Could you check a few things on this model? Use its own coordinates, in mm. A direction names the side the tool comes from. Coordinates: 2 decimals unless noted, no trailing zeros. Loops run counter-clockwise (first coordinate to the right, second up) from the corner with the lowest first, then second, coordinate; pieces in that order, holes last. Notation, with made-up numbers: (88.25, 37.25) - (117.25, 37.25) arc R16 ccw to (117.25, 65.25) - close; hole circle Ø1 at (-12, 43). An arc over 180 degrees is marked (long way). Use CSV: the item, a comma, the result in double quotes.
from build123d import *

# Parameters (mm, degrees)
BOSS_EXTRUDE1_START     = -26
SKETCH1_R               = 20
BOSS_EXTRUDE1_DEPTH     = 3
BOSS_EXTRUDE2_START     = -26
SKETCH2_W               = 20
SKETCH2_H               = 49
BOSS_EXTRUDE2_DEPTH     = 3
BOSS_EXTRUDE3_START     = -26
SKETCH3_W               = 3
SKETCH3_H               = 49
BOSS_EXTRUDE3_DEPTH     = 38
CUT_EXTRUDE1_DEPTH      = 52.730068626
CUT_EXTRUDE1_DEPTH_BACK = 52.730068626
SKETCH4_R               = 2.75
SKETCH4_R_2             = 0.8
CUT_EXTRUDE2_DEPTH      = 52.730068626
CUT_EXTRUDE2_DEPTH_BACK = 52.730068626
SKETCH5_R               = 1.725


with BuildPart() as part:
    # Sketch1 → Boss-Extrude1 (new body)
    with BuildSketch(Plane.XY.offset(BOSS_EXTRUDE1_START)):
        Circle(SKETCH1_R)
    extrude(amount=BOSS_EXTRUDE1_DEPTH)

    # Sketch2 → Boss-Extrude2 (add)
    with BuildSketch(Plane.XY.offset(BOSS_EXTRUDE2_START)):
        with Locations((10, -15.5)):
            Rectangle(SKETCH2_W, SKETCH2_H)
    extrude(amount=BOSS_EXTRUDE2_DEPTH)

    # Sketch3 → Boss-Extrude3 (add)
    with BuildSketch(Plane.XY.offset(BOSS_EXTRUDE3_START)):
        with Locations((18.5, -15.5)):
            Rectangle(SKETCH3_W, SKETCH3_H)
    extrude(amount=BOSS_EXTRUDE3_DEPTH)

    # Sketch4 → Cut-Extrude1 (cut, two sides: drawn at the far end of the back side and taken through both)
    with BuildSketch(Plane.XY.offset(-CUT_EXTRUDE1_DEPTH_BACK)):
        Circle(SKETCH4_R)
        with Locations((0, 6)):
            Circle(SKETCH4_R_2)
        with Locations((0, -6)):
            Circle(SKETCH4_R_2)
        with Locations((0, 17)):
            Circle(SKETCH4_R_2)
        with Locations((0, -17)):
            Circle(SKETCH4_R_2)
    extrude(amount=CUT_EXTRUDE1_DEPTH + CUT_EXTRUDE1_DEPTH_BACK, mode=Mode.SUBTRACT)

    # Sketch5 → Cut-Extrude2 (cut, two sides: drawn at the far end of the back side and taken through both)
    with BuildSketch(Plane(origin=(0, 0, 0), x_dir=(0, 0, -1), z_dir=(1, 0, 0)).offset(-CUT_EXTRUDE2_DEPTH_BACK)):
        with Locations((-6, -31)):
            Circle(SKETCH5_R)
        with Locations((6, -31)):
            Circle(SKETCH5_R)
    extrude(amount=CUT_EXTRUDE2_DEPTH + CUT_EXTRUDE2_DEPTH_BACK, mode=Mode.SUBTRACT)


solid = part.part
(1) Suppose I cut it at A-A (y = 0). Write out the boundary of the cut face in (x, z), plus the area to 4 significant figures.
Computed:
outline,"(-20, -26) - (-2.75, -26) - (-2.75, -23) - (-20, -23) - close; (2.75, -26) - (20, -26) - (20, 12) - (17, 12) - (17, -23) - (2.75, -23) - close"
area,"208.5 mm²"
(2) Thinking about a two-plate mould opening in Z: for faces 1 (the face through (4, -10, -26)), 2 (the face through (0.37, 16.29, -24.52)), 3 (the face through (18.479, -32.684, -5.626)), which applies, +Z half, -Z half, draft (parallel to the pull), parting line (faces both ways), or undercut?
Computed:
face 1,"-Z half"
face 2,"draft"
face 3,"undercut"
(3) Suppose I cut it at C-C (y = -31). Write out the boundary of the cut face in (x, z) (3 decimals), plus the area to 3 significant figures.
Computed:
outline,"(0, -26) - (20, -26) - (20, -7.725) - (17, -7.725) - (17, -23) - (0, -23) - close; (17, -4.275) - (20, -4.275) - (20, 4.275) - (17, 4.275) - close; (17, 7.725) - (20, 7.725) - (20, 12) - (17, 12) - close"
area,"144 mm²"
(4) Please list where these lines run through material, in increasing order: line 1 (Z direction, x = 18, y = -31) (3 decimals); line 2 (X direction, y = 0, z = -24); line 3 (Y direction, x = 18, z = -6) (3 decimals).
Computed:
line 1,"z = -26 to -7.725, -4.275 to 4.275, 7.725 to 12"
line 2,"x = -20 to -2.75, 2.75 to 20"
line 3,"y = -40 to -32.725, -29.275 to 9"
(5) Suppose I cut it at D-D (x = 16). Write out the boundary of the cut face in (y, z).
Computed:
outline,"(-40, -26) - (12, -26) - (12, -23) - (-40, -23) - close"
(6) Will these pins go through, and if not, where does the flat tip stop? pin 1 (12 mm diameter, centred on y = -25.5, z = -10.5, fed in from -X); pin 2 (2 mm diameter, centred on x = 0, y = 6, fed in from +Z); pin 3 (1.5 mm diameter, centred on y = -26, z = -25, fed in from -X).
Computed:
pin 1,"stops at x = 17"
pin 2,"stops at z = -23"
pin 3,"stops at x = 0"
(7) Which directions (+Z, -Z, +X, -X, +Y, -Y) give clear straight access to the entire face, cutting with the end or side of a thin tool? Please do faces 4 (the face through (0, -30, -25)), 5 (the face through (0.37, -17.71, -24.52)), 6 (the face through (17, -16, -6)).
Computed:
face 4,"+Z, -Z, -X, -Y"
face 5,"+Z, -Z"
face 6,"+Z, -X, +Y, -Y"
(8) Suppose I cut it at B-B (z = 6). Write out the boundary of the cut face in (x, y) (3 decimals), plus the area to 3 significant figures.
Computed:
outline,"(17, -40) - (20, -40) - (20, -32.725) - (17, -32.725) - close; (17, -29.275) - (20, -29.275) - (20, 9) - (17, 9) - close"
area,"137 mm²"
